For this review, use the dimensioned drawing (mm, ordinates from the lowest corner) and the shaded views. A direction names the side the tool comes from. Give positions to 0.01 mm unless a question says otherwise; leave off trailing zeros. Loops run counter-clockwise (first coordinate to the right, second up) from the corner with the lowest first, then second, coordinate; pieces in that order, holes last. Notation, with made-up numbers: M 69,6 L 93,6 A6 cw 93,15 Z; hole C -22.5,68.25 d4. An arc over 180 degrees is marked long. Use CSV: the item, a comma, the result in double quotes. Start each with the question number.
1. Take a section at D-D, the plane y = 21. Write out the cut boundary in (x, z), and give its area (3 significant figures).
2. Take a section at C-C, the plane z = 8. Write out the cut boundary in (x, y).
3. Take a section at A-A, the plane x = 5. Write out the cut boundary in (y, z).
4. To check wall thickness, follow line 1 (Z direction, x = 45.6, y = 26); line 2 (Y direction, x = 5, z = 1); line 3 (Y direction, x = 46, z = 42). State the ranges of each line that lie inside material, in increasing order. Write a range as [from, to].
5. Take a section at B-B, the plane y = 5. Write out the cut boundary in (x, z).
6. Insertion check: P1, Ø2.5, axis at x = 17.5, y = 26, coming from the +Z side; P2, Ø8, axis at y = 27, z = 21, coming from the -X side; P3, Ø2, axis at y = 26, z = 8, coming from the -X side. Each pin has a flat end and moves straight along its axis. Give the tip position at first contact, or say it passes through.
7. Tool access review of the marked faces 1 and 2: name each direction out of +Z, -Z, +X, -X, +Y, -Y from which nothing blocks a thin tool from reaching the whole face with its end or side.
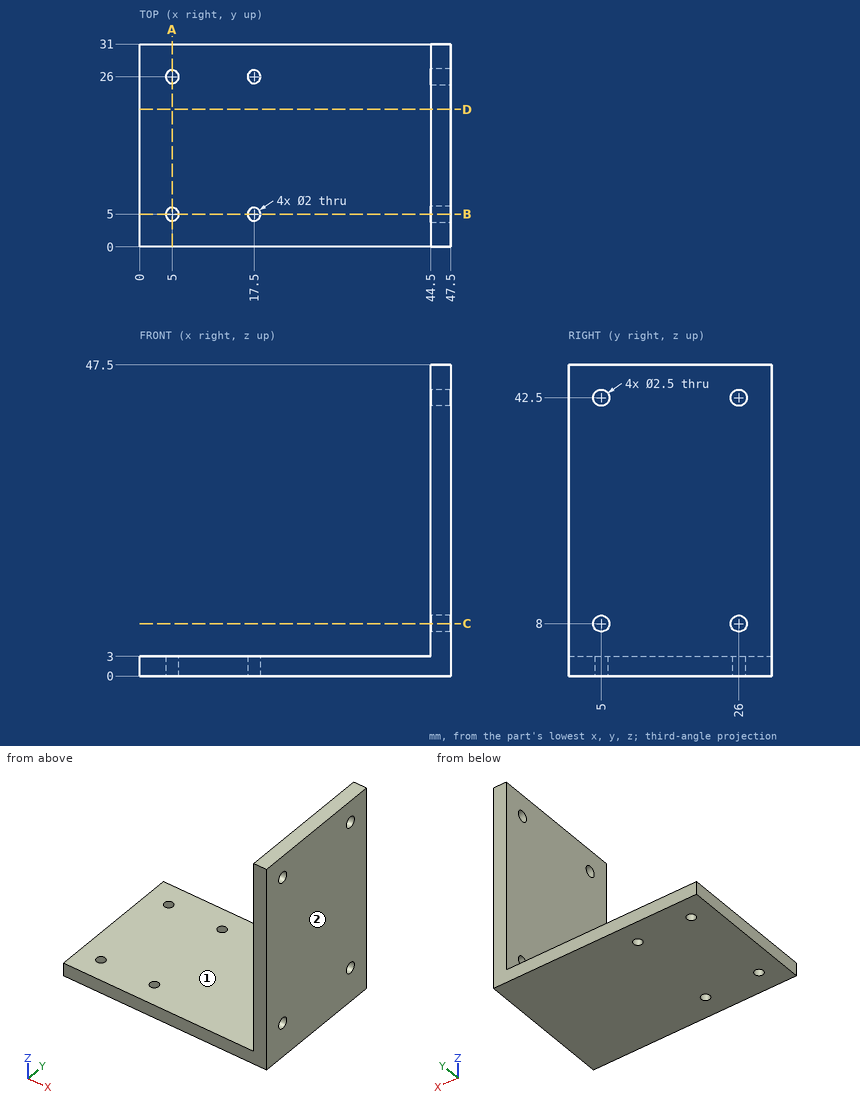
Result set:
1,outline,"M 0,0 L 47.5,0 L 47.5,47.5 L 44.5,47.5 L 44.5,3 L 0,3 Z"
1,area,"276 mm2"
2,outline,"M 44.5,0 L 47.5,0 L 47.5,3.75 L 44.5,3.75 Z; M 44.5,6.25 L 47.5,6.25 L 47.5,24.75 L 44.5,24.75 Z; M 44.5,27.25 L 47.5,27.25 L 47.5,31 L 44.5,31 Z"
3,outline,"M 0,0 L 4,0 L 4,3 L 0,3 Z; M 6,0 L 25,0 L 25,3 L 6,3 Z; M 27,0 L 31,0 L 31,3 L 27,3 Z"
4,line 1,"[0, 6.75], [9.25, 41.25], [43.75, 47.5]"
4,line 2,"[0, 4], [6, 25], [27, 31]"
4,line 3,"[0, 3.85], [6.15, 24.85], [27.15, 31]"
5,outline,"M 0,0 L 4,0 L 4,3 L 0,3 Z; M 6,0 L 16.5,0 L 16.5,3 L 6,3 Z; M 18.5,0 L 47.5,0 L 47.5,6.75 L 44.5,6.75 L 44.5,3 L 18.5,3 Z; M 44.5,9.25 L 47.5,9.25 L 47.5,41.25 L 44.5,41.25 Z; M 44.5,43.75 L 47.5,43.75 L 47.5,47.5 L 44.5,47.5 Z"
6,P1,"z = 3"
6,P2,"x = 44.5"
6,P3,"through"
7,face 1,"+Z, -X, +Y, -Y"
7,face 2,"+Z, -Z, +X, +Y, -Y"
